```python
from build123d import *

# Parameters (mm, degrees)
SKETCH_1_W          = 10
SKETCH_1_H          = 12
SKETCH_2_R          = 4.3
AXIAL_BORE_DEPTH    = 19.547236991
SKETCH_3_R          = 8.3
D16_CLEARANCE_DEPTH = 19.547236991


with BuildPart() as part:
    # 草图1 → Round_pushrod_head (revolve)
    with BuildSketch(Plane.XY, mode=Mode.PRIVATE) as round_pushrod_head_sk:
        with Locations((5, 6)):
            Rectangle(SKETCH_1_W, SKETCH_1_H)
    revolve(round_pushrod_head_sk.sketch.rotate(Axis((0, 0, 0), (0, 1, 0)), 90), axis=Axis((0, 0, 0), (0, 1, 0)))

    # 草图2 → Axial_bore (cut, through all)
    with BuildSketch(Plane(origin=(0, 12, 0), x_dir=(1, 0, 0), z_dir=(0, 1, 0))):
        with Locations(Location((0, 0, 0), (0, 0, 270))):
            Circle(SKETCH_2_R)
    extrude(amount=-AXIAL_BORE_DEPTH, mode=Mode.SUBTRACT)

    # 草图3 → D16_clearance (cut, through all)
    with BuildSketch(Plane(origin=(0, 12, 0), x_dir=(1, 0, 0), z_dir=(0, 1, 0))):
        with Locations(Location((0, 0, 0), (0, 0, 270))):
            Circle(SKETCH_3_R)
    extrude(amount=-D16_CLEARANCE_DEPTH, mode=Mode.SUBTRACT)


solid = part.part
```
Geometry check sheet. Reference: the model listing, model coordinates, mm. Round coordinates to 2 decimals unless told otherwise and drop trailing zeros. Loops run counter-clockwise (first coordinate to the right, second up) from the corner with the lowest first, then second, coordinate; pieces in that order, holes last. Notation, with made-up numbers: (63, 73.5) - (122, 73.5) arc R17 cw to (122, 81.5) - close; hole circle Ø8 at (14, -33). An arc over 180 degrees is marked (long way). Write each question's results on one line, items separated by ' | '. Start each with the question number.
Q1. Cross-section at A-A on x = 0. Enter the section's corners in (y, z).
Q2. Release check for a two-part mould opening along Z. For faces 1 (the cylindrical face through (0, 6, 10)), 2 (the cylindrical face through (-5.05, 6.084, -6.587)), 3 (the flat face through (-6, 0, -6)) record: +Z half, -Z half, draft (parallel to the pull), parting line (faces both ways), or undercut.
Q3. Cross-section at C-C on y = 2.5. Enter the section's corners in (x, z).
Q4. Gauge pin test, flat ends, axial feed: P1, Ø1, axis at x = -7.5, y = 5.5, coming from the +Z side; P2, Ø5, axis at x = -5, y = 9, coming from the +Z side; P3, Ø5, axis at x = -6, z = -5, coming from the +Y side; P4, Ø1, axis at x = -3.5, y = 6, coming from the -Z side. Record the tip position at first contact, or that the pin passes through.
Q5. Thickness scan on line 1 (X direction, y = 9.25, z = 0); line 2 (X direction, y = 6.75, z = -3.5); line 3 (Z direction, x = 8.75, y = 9.25). Record the ranges inside material, lowest first. Write a range as [from, to].
Q6. Cross-section at B-B on z = 0. Enter the section's corners in (x, y).
Answers below:
1) outline: (0, -10) - (12, -10) - (12, -8.3) - (0, -8.3) - close; (0, 8.3) - (12, 8.3) - (12, 10) - (0, 10) - close
2) face 1: parting line | face 2: undercut | face 3: draft
3) outline: circle Ø20 at (0, 0); hole circle Ø16.6 at (0, 0)
4) P1: stops at z = 7.14 | P2: stops at z = 9.68 | P3: stops at y = 12 | P4: stops at z = -9.54
5) line 1: x = [-10, -8.3], [8.3, 10] | line 2: x = [-9.37, -7.53], [7.53, 9.37] | line 3: z = [-4.84, 4.84]
6) outline: (-10, 0) - (-8.3, 0) - (-8.3, 12) - (-10, 12) - close; (8.3, 0) - (10, 0) - (10, 12) - (8.3, 12) - close
